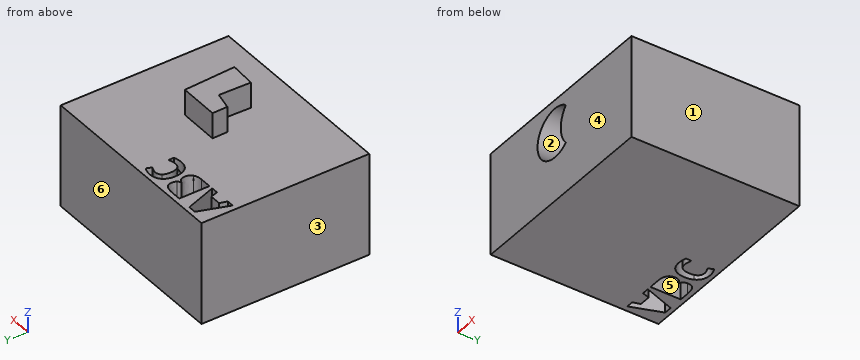
from build123d import *

# Parameters (mm, degrees)
F0_W     = 99.7463464737
F0_H     = 83.5314244032
F1_DEPTH = 50.8
F3_DEPTH = 76.2
F5_DEPTH = 12.7


with BuildPart() as f1:
    # F0 (on Top) → F1 (new body)
    with BuildSketch(Plane.XY):
        with Locations((4.4222511351, -4.3403580785)):
            Rectangle(F0_W, F0_H)
        Polygon((-28.2221282138, 20.0006692662), (-31.6609589625, 20.0006692662), (-32.7512395926, 23.5844315791), (-38.2388756342, 23.5844315791), (-39.3291562643, 20.0006692662), (-42.767987013, 20.0006692662), (-37.4549276283, 35.1130787253), (-33.5549509937, 35.1130787253), align=None, mode=Mode.SUBTRACT)
        with BuildLine():
            Line((-26.3281361826, 20.0006692662), (-26.3281361826, 35.0504946407))
            Line((-26.3281361826, 35.0504946407), (-21.6442115421, 35.0504946407))
            add(Edge.make_bspline(
                [(-21.6442115421, 35.0504946407), (-18.4425415347, 35.0504946407), (-16.9965197926, 34.1397315162)],
                knots=[0, 0, 0, 1, 1, 1], degree=2))
            add(Edge.make_bspline(
                [(-16.9965197926, 34.1397315162), (-15.5504980506, 33.2289683917), (-15.5504980506, 31.2427471833)],
                knots=[0, 0, 0, 1, 1, 1], degree=2))
            add(Edge.make_bspline(
                [(-15.5504980506, 31.2427471833), (-15.5504980506, 29.8922485176), (-16.182926694, 29.0275999817)],
                knots=[0, 0, 0, 1, 1, 1], degree=2))
            add(Edge.make_bspline(
                [(-16.182926694, 29.0275999817), (-16.8153553375, 28.1629514457), (-17.8661091773, 27.9883747889)],
                knots=[0, 0, 0, 1, 1, 1], degree=2))
            Line((-17.8661091773, 27.9883747889), (-17.8661091773, 27.8862639142))
            add(Edge.make_bspline(
                [(-17.8661091773, 27.8862639142), (-16.4365569312, 27.5667556933), (-15.8024813382, 26.6922254598)],
                knots=[0, 0, 0, 1, 1, 1], degree=2))
            add(Edge.make_bspline(
                [(-15.8024813382, 26.6922254598), (-15.1684057452, 25.8176952263), (-15.1684057452, 24.3650856859)],
                knots=[0, 0, 0, 1, 1, 1], degree=2))
            add(Edge.make_bspline(
                [(-15.1684057452, 24.3650856859), (-15.1684057452, 22.3063986955), (-16.6572481766, 21.1535339809)],
                knots=[0, 0, 0, 1, 1, 1], degree=2))
            add(Edge.make_bspline(
                [(-16.6572481766, 21.1535339809), (-18.146090608, 20.0006692662), (-20.6988624761, 20.0006692662)],
                knots=[0, 0, 0, 1, 1, 1], degree=2))
            Line((-20.6988624761, 20.0006692662), (-26.3281361826, 20.0006692662))
        make_face(mode=Mode.SUBTRACT)
        with BuildLine():
            add(Edge.make_bspline(
                [(-4.0943166865, 32.3116174687), (-4.9474365753, 32.6097153449), (-5.7709113714, 32.6097153449)],
                knots=[0, 0, 0, 1, 1, 1], degree=2))
            add(Edge.make_bspline(
                [(-5.7709113714, 32.6097153449), (-7.5726742254, 32.6097153449), (-8.5608439808, 31.2559227801)],
                knots=[0, 0, 0, 1, 1, 1], degree=2))
            add(Edge.make_bspline(
                [(-8.5608439808, 31.2559227801), (-9.5490137362, 29.9021302152), (-9.5490137362, 27.4844082137)],
                knots=[0, 0, 0, 1, 1, 1], degree=2))
            add(Edge.make_bspline(
                [(-9.5490137362, 27.4844082137), (-9.5490137362, 22.4513302596), (-5.7709113714, 22.4513302596)],
                knots=[0, 0, 0, 1, 1, 1], degree=2))
            add(Edge.make_bspline(
                [(-5.7709113714, 22.4513302596), (-4.1865458636, 22.4513302596), (-1.9335188214, 23.2418660639)],
                knots=[0, 0, 0, 1, 1, 1], degree=2))
            Line((-1.9335188214, 23.2418660639), (-1.9335188214, 20.567219926))
            add(Edge.make_bspline(
                [(-1.9335188214, 20.567219926), (-3.7846901631, 19.7931536176), (-6.0706561972, 19.7931536176)],
                knots=[0, 0, 0, 1, 1, 1], degree=2))
            add(Edge.make_bspline(
                [(-6.0706561972, 19.7931536176), (-9.3546736843, 19.7931536176), (-11.0938524538, 21.7859626243)],
                knots=[0, 0, 0, 1, 1, 1], degree=2))
            add(Edge.make_bspline(
                [(-11.0938524538, 21.7859626243), (-12.8330312233, 23.778771631), (-12.8330312233, 27.5041716088)],
                knots=[0, 0, 0, 1, 1, 1], degree=2))
            add(Edge.make_bspline(
                [(-12.8330312233, 27.5041716088), (-12.8330312233, 29.8527217274), (-11.9782643849, 31.6182516904)],
                knots=[0, 0, 0, 1, 1, 1], degree=2))
            add(Edge.make_bspline(
                [(-11.9782643849, 31.6182516904), (-11.1234975464, 33.3837816533), (-9.5226625427, 34.3241898705)],
                knots=[0, 0, 0, 1, 1, 1], degree=2))
            add(Edge.make_bspline(
                [(-9.5226625427, 34.3241898705), (-7.921827539, 35.2645980877), (-5.7709113714, 35.2645980877)],
                knots=[0, 0, 0, 1, 1, 1], degree=2))
            add(Edge.make_bspline(
                [(-5.7709113714, 35.2645980877), (-3.5804684137, 35.2645980877), (-1.3669681616, 34.2072564495)],
                knots=[0, 0, 0, 1, 1, 1], degree=2))
            Line((-1.3669681616, 34.2072564495), (-2.3946647072, 31.611663892))
            add(Edge.make_bspline(
                [(-2.3946647072, 31.611663892), (-3.2411967977, 32.0135195925), (-4.0943166865, 32.3116174687)],
                knots=[0, 0, 0, 1, 1, 1], degree=2))
        make_face(mode=Mode.SUBTRACT)
    extrude(amount=F1_DEPTH)

    # F2 (on face) → F3 (cut)
    with BuildSketch(Plane.XZ.offset(46.1060702801)):
        with BuildLine():
            ThreePointArc((7.7817309512, 24.7494648312), (4.2001656167, 34.2502631247), (7.7817309512, 43.7510614182))
            ThreePointArc((7.7817309512, 43.7510614182), (-12.2809, 34.2502631247), (7.7817309512, 24.7494648312))
        make_face()
    extrude(amount=-F3_DEPTH, mode=Mode.SUBTRACT)

    # F4 (on face) → F5 (join)
    with BuildSketch(Plane.XY.offset(50.8)):
        Polygon((19.7219643742, -0.1289248466), (0, 0), (0.1093503088, -7.4666291475), (8.8314060122, -9.341686964), (8.3788465708, -25.0158682466), (21.0125762969, -25.6724208593), align=None)
    extrude(amount=F5_DEPTH)


solid = f1.part
Design review of the part built by this model. Coordinates are the model's own, in mm. Face numbers are marked on the shaded views. A direction names the side the tool comes from. Give positions to 0.01 mm unless a question says otherwise; leave off trailing zeros. Loops run counter-clockwise (first coordinate to the right, second up) from the corner with the lowest first, then second, coordinate; pieces in that order, holes last. Notation, with made-up numbers: M -18,13.25 L 29,13.25 A19 ccw 29,48.25 Z; hole C 78.5,54.25 d8. An arc over 180 degrees is marked long. Answer as a JSON object with one key per item and string values.
Item 1: Machinability: for the marked faces 1 and 2, which of the approach directions +Z, -Z, +X, -X, +Y, -Y give a long, thin tool a straight path to every point of the face, cutting with its end or side? Answer none if there is none.
Output values:
{"face 1": "+Z, -Z, +X, +Y, -Y", "face 2": "-Y"}
Item 2: For P1, Ø1, axis at x = 22, y = -2, coming from the +Z side, flat-tipped, find the tip position at first contact; note if it passes through.
Output values:
{"P1": "stops at z = 50.8"}
Item 3: We need section D-D (z = 58). State the section outline as (x, y) points, and give its area (3 significant figures).
Output values:
{"outline": "M 0,0 L 0.11,-7.47 L 8.83,-9.34 L 8.38,-25.02 L 21.01,-25.67 L 19.72,-0.13 Z", "area": "368 mm2"}
Item 4: Mouldability with a two-part tool opening along Y and no side actions: class the marked faces 3, 4, 5 and 6 as pulls with the +Y half, pulls with the -Y half, needs draft (parallel to the pull), parting line crosses it, or undercut.
Output values:
{"face 3": "needs draft", "face 4": "pulls with the -Y half", "face 5": "undercut", "face 6": "pulls with the +Y half"}
Item 5: We need section A-A (y = 8). State the section outline as (x, z) points, and give its area (3 significant figures).
Output values:
{"outline": "M -45.45,0 L 54.3,0 L 54.3,50.8 L -45.45,50.8 Z; hole M 7.78,24.75 A14.39 cw 7.78,43.75 A12.28 ccw long Z", "area": "4,700 mm2"}
Item 6: Wall thickness on line 1 along Z through (x, y) = (6.5, -4); line 2 along Y through (x, z) = (-37, 33.5); line 3 along Z through (x, y) = (0, 8): over which ranges is each line inside the solid? List them lowest first.
Output values:
{"line 1": "z = 0 to 23.83, 26.45 to 42.05, 44.67 to 63.5", "line 2": "y = -46.11 to 23.58, 35.11 to 37.43", "line 3": "z = 0 to 21.97, 46.53 to 50.8"}
Item 7: We need section B-B (z = 14.5). Count the separate pieces of the cut face and the enclosed holes in it, and give its area (3 significant figures).
Output values:
{"separate pieces": "1", "enclosed holes": "3", "area": "7,980 mm2"}
